Could you check a few things on this model? Use its own coordinates, in mm. A direction names the side the tool comes from. Round coordinates to 2 decimals unless told otherwise and drop trailing zeros. Write each loop counter-clockwise with the first axis right and the second up, starting at its lowest first coordinate (ties: lowest second). Pieces come first, ordered by that corner, then holes. Notation, with made-up numbers: (34.5, -31) -> (47.5, -31) arc R27 ccw to (47.5, -13) -> close; hole circle Ø1 at (64, -7). An arc over 180 degrees is marked (long way). Answer in a Markdown table with one row per item.
Autodesk Inventor part; units mm, degrees
ref_plane "YZ Plane" through (0, 0, 0) normal (1, 0, 0) x (0, 1, 0)
ref_plane "XZ Plane" through (0, 0, 0) normal (0, 1, 0) x (-1, 0, 0)
ref_plane "XY Plane" through (0, 0, 0) normal (0, 0, 1) x (1, 0, 0)
sketch "Sketch1" plane through (0, 0, 0) normal (0, 0, 1) x (1, 0, 0)
  line L0 (0, 0) -> (0, 12.7)
  line L1 (0, 12.7) -> (12.7, 12.7)
  line L2 (12.7, 12.7) -> (12.7, 11.43)
  line L3 (12.7, 11.43) -> (1.27, 11.43)
  line L4 (1.27, 11.43) -> (1.27, 0)
  line L5 (1.27, 0) -> (0, 0)
  dimension "d0" = 12.7
  dimension "d1" = 12.7
  dimension "d2" = 1.27
  dimension "d3" = 11.43
extrude "Extrusion1" add sketch "Sketch1" along normal blind 292.1
sketch "Sketch3" plane through (0, 12.7, 0) normal (0, 1, 0) x (1, 0, 0)
  line L0 (12.7, -292.1) -> (0, -292.1)
  line L1 (12.7, 0) -> (12.7, -292.1)
  line L2 (0, -292.1) -> (12.7, -279.4)
  dimension "d10" = 45
extrude "Extrusion3" cut sketch "Sketch3" against normal blind 25.4
properties part number "Aluminum Angle 3 Left" material "Aluminum 6061"
1) Please list where these lines run through material, in increasing order: line 1 (Y direction, x = 5.75, z = 84.5); line 2 (X direction, y = 5, z = 23.5); line 3 (Z direction, x = 10.25, y = 12).
Findings:
| item | result |
|---|---|
| line 1 | y = 11.43 to 12.7 |
| line 2 | x = 0 to 1.27 |
| line 3 | z = 0 to 281.85 |
2) Imagine slicing it at A-A, the plane z = 132. Please give me the cut outline in (x, y), plus the area to 3 significant figures.
Findings:
| item | result |
|---|---|
| outline | (0, 0) -> (1.27, 0) -> (1.27, 11.43) -> (12.7, 11.43) -> (12.7, 12.7) -> (0, 12.7) -> close |
| area | 30.6 mm^2 |
3) For faces 1 (the face through (3.5, 11.6, 288.6)), 2 (the face through (7, 11.43, 143)), which set-ups out of +Z, -Z, +X, -X, +Y, -Y let a thin tool reach every point of the face, with its end or its side?
Findings:
| item | result |
|---|---|
| face 1 | +Z, +X, +Y, -Y |
| face 2 | +Z, -Z, +X, -Y |
4) For pin 1 (2 mm diameter, centred on y = 3.5, z = 142.5, fed in from +X); pin 2 (1.5 mm diameter, centred on x = 3, z = 193.5, fed in from -Y); pin 3 (5 mm diameter, centred on y = 6.5, z = 56.5, fed in from -X), each with a flat end and sliding along its axis, tell me the tip position at first contact or that it passes through.
Findings:
| item | result |
|---|---|
| pin 1 | stops at x = 1.27 |
| pin 2 | stops at y = 11.43 |
| pin 3 | stops at x = 0 |
5) Imagine slicing it at B-B, the plane x = 5. Please give me the cut outline in (y, z), plus the area to 3 significant figures.
Findings:
| item | result |
|---|---|
| outline | (11.43, 0) -> (12.7, 0) -> (12.7, 287.1) -> (11.43, 287.1) -> close |
| area | 365 mm^2 |
6) Imagine slicing it at C-C, the plane y = 7. Please give me the cut outline in (x, z).
Findings:
| item | result |
|---|---|
| outline | (0, 0) -> (1.27, 0) -> (1.27, 290.83) -> (0, 292.1) -> close |
